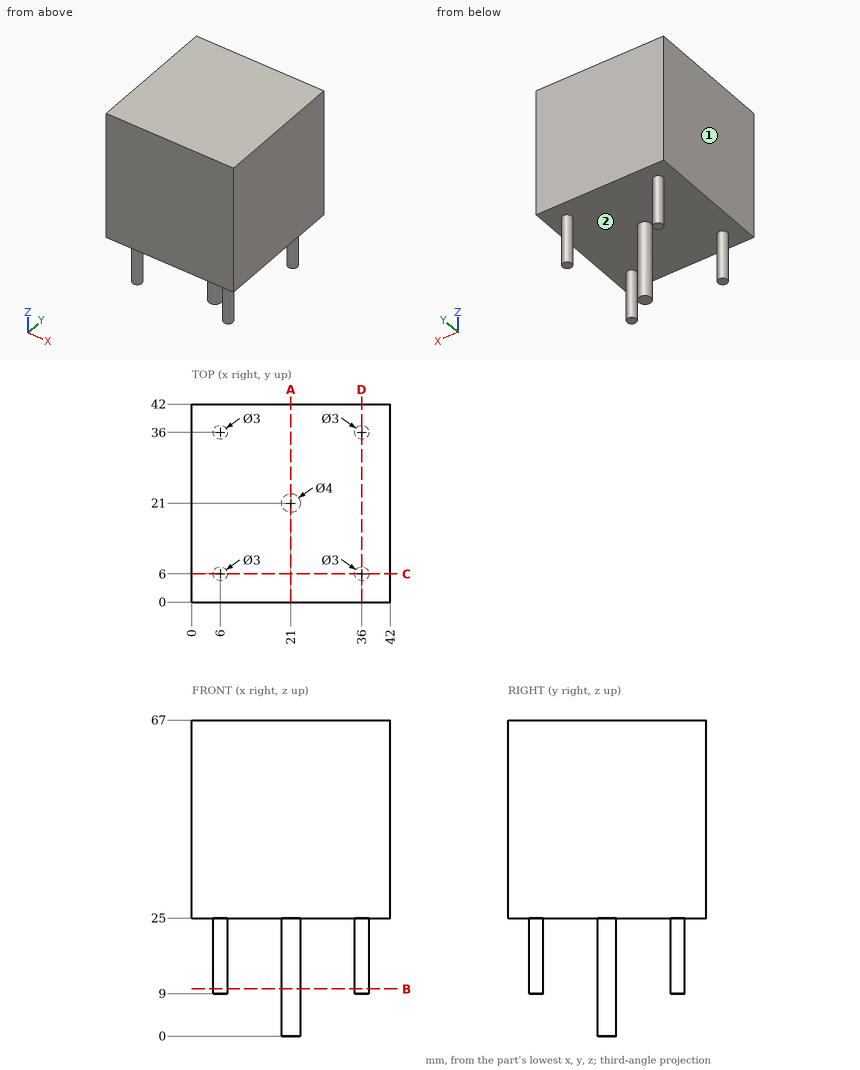
Source: three-view drawing plus pictorial views. Frame: mm from the lowest corner of the part. A direction names the side the tool comes from. Coordinates: 2 decimals unless noted, no trailing zeros. Order: outer loops, then holes, each group sorted by start corner. A loop starts at its lowest first (then second) coordinate and runs counter-clockwise, first axis right, second up.
Item 1: Set-up query: the marked faces 1 and 2. Return all of +Z, -Z, +X, -X, +Y, -Y with unobstructed straight access to the full face (end or side cutting, diameter ignored); none if empty.
Output values:
face 1: +Z, -Z, -X, +Y, -Y
face 2: -Z
Item 2: Material intervals for line 1 (X direction, y = 36, z = 19); line 2 (Y direction, x = 35.5, z = 23.5); line 3 (Z direction, x = 17, y = 23), sorted ascending.
Output values:
line 1: x = 4.5 to 7.5, 34.5 to 37.5
line 2: y = 4.59 to 7.41, 34.59 to 37.41
line 3: z = 25 to 67
Item 3: First-contact query: P1, Ø2.5, axis at x = 35.5, y = 6, coming from the -Z side; P2, Ø1, axis at x = 15, y = 37, coming from the -Z side. Flat tips, straight axial feed; report the tip coordinate or a pass-through.
Output values:
P1: stops at z = 9
P2: stops at z = 25
Item 4: Cut plane C-C (y = 6). Return loops of the section in (x, z).
Output values:
outline: (0, 25) - (4.5, 25) - (4.5, 9) - (7.5, 9) - (7.5, 25) - (34.5, 25) - (34.5, 9) - (37.5, 9) - (37.5, 25) - (42, 25) - (42, 67) - (0, 67) - close
Item 5: Cut plane B-B (z = 10). Return loops of the section in (x, y), plus the area to 3 significant figures.
Output values:
outline: circle Ø3 at (6, 6); circle Ø3 at (6, 36); circle Ø4 at (21, 21); circle Ø3 at (36, 6); circle Ø3 at (36, 36)
area: 40.8 mm2
Item 6: Cut plane A-A (x = 21). Return loops of the section in (y, z).
Output values:
outline: (0, 25) - (19, 25) - (19, 0) - (23, 0) - (23, 25) - (42, 25) - (42, 67) - (0, 67) - close
